from build123d import *

# Parameters (mm, degrees)
F0_W     = 15
F0_H     = 14
F0_R     = 3
F0_W_2   = 20
F0_H_2   = 2
F1_DEPTH = 2
F0_H_3   = 28
F0_W_3   = 12.9
F0_H_4   = 19.9
F2_DEPTH = 11.25
F3_R     = 5
F4_W     = 2
F4_H     = 1
F5_DEPTH = 2
F6_R     = 4.5
F6_R_2   = 2.75
F7_DEPTH = 9.25
F8_DEPTH = 2.001


with BuildPart() as f1:
    # F0 (on Top) → F1 (new body)
    with BuildSketch(Plane.XY):
        with Locations((-0.1896551724, 11.6551724138)):
            Rectangle(F0_W, F0_H)
        with Locations((-0.1896551724, 11.6551724138)):
            Circle(F0_R, mode=Mode.SUBTRACT)
        Polygon((-7.6896551724, 4.6551724138), (-22.6896551724, 4.6551724138), (-22.6896551724, 0.6551724138), (-9.1896551724, 0.6551724138), (10.8103448276, 0.6551724138), (24.3103448276, 0.6551724138), (24.3103448276, 4.6551724138), (7.3103448276, 4.6551724138), align=None)
        Polygon((-9.1896551724, 0.6551724138), (-22.6896551724, 0.6551724138), (-22.6896551724, -29.3448275862), (-9.1896551724, -29.3448275862), (-9.1896551724, -27.3448275862), align=None)
        Polygon((24.3103448276, 0.6551724138), (10.8103448276, 0.6551724138), (10.8103448276, -27.3448275862), (10.8103448276, -29.3448275862), (24.3103448276, -29.3448275862), align=None)
        with Locations((0.8103448276, -28.3448275862)):
            Rectangle(F0_W_2, F0_H_2)
    extrude(amount=F1_DEPTH)

    # F0 (on Top) → F2 (join)
    with BuildSketch(Plane.XY):
        with Locations((0.8103448276, -13.3448275862)):
            Rectangle(F0_W_2, F0_H_3)
        with Locations((0.8103448276, -15.3448275862)):
            Rectangle(F0_W_3, F0_H_4, mode=Mode.SUBTRACT)
    extrude(amount=F2_DEPTH)

    # F3
    f3_edges = [f1.edges().sort_by_distance(p)[0] for p in [
        (10.810345, 0.655172, 6.625),
        (-9.189655, 0.655172, 6.625),
        (-9.189655, -27.344828, 6.625),
        (10.810345, -27.344828, 6.625),
        (24.310345, -29.344828, 1),
        (-22.689655, -29.344828, 1),
        (24.310345, 4.655172, 1),
        (7.310345, 18.655172, 1),
        (-7.689655, 18.655172, 1),
        (-22.689655, 4.655172, 1),
        (-7.689655, 4.655172, 1),
        (7.310345, 4.655172, 1),
    ]]
    fillet(f3_edges, radius=F3_R)

    # F4 (on face) → F5 (cut)
    with BuildSketch(Plane(origin=(0, 0, 0), x_dir=(1, 0, 0), z_dir=(0, 0, -1))):
        with Locations((0.8603448276, 25.7948275862)):
            Rectangle(F4_W, F4_H)
        with Locations((0.8603448276, 4.8948275862)):
            Rectangle(F4_W, F4_H)
    extrude(amount=-F5_DEPTH, mode=Mode.SUBTRACT)

    # F6 (on face) → F7 (join)
    with BuildSketch(Plane.XY.offset(2)):
        with Locations((-15.6896551724, -23.3448275862)):
            Circle(F6_R)
        with Locations((-15.6896551724, -23.3448275862)):
            Circle(F6_R_2, mode=Mode.SUBTRACT)
        with Locations((17.3103448276, -23.3448275862)):
            Circle(F6_R)
        with Locations((17.3103448276, -23.3448275862)):
            Circle(F6_R_2, mode=Mode.SUBTRACT)
    extrude(amount=F7_DEPTH)

    # F8 (cut, through all): faces of the model
    f8_faces = [f1.faces().sort_by_distance(p)[0] for p in [
        (-15.6896551724, -23.3448275862, 2),
        (17.3103448276, -23.3448275862, 2),
    ]]
    extrude(f8_faces, amount=-F8_DEPTH, mode=Mode.SUBTRACT)


solid = f1.part
Build history of the part. All positions in model axes, mm. A direction names the side the tool comes from. Coordinates: 2 decimals unless noted, no trailing zeros. Order: outer loops, then holes, each group sorted by start corner. A loop starts at its lowest first (then second) coordinate and runs counter-clockwise, first axis right, second up. Notation, with made-up numbers: (44, 32) - (64, 32) arc R10 ccw to (64, 47) - close; hole circle Ø4 at (40.5, 16.25). An arc over 180 degrees is marked (long way). Write item = value, one per line. Start each with the question number.
1) Wall check: line 1 along X through (y, z) = (-7, 7); line 2 along X through (y, z) = (-15, 0.75); line 3 along X through (y, z) = (-23.5, 8.5). Give the ranges that are in metal, low to high. Write a range as from..to.
2) Saw through at B-B on y = -12.5. Write the cut outline in (x, z), then the cut area to 3 significant figures.
3) Saw through at A-A on z = 4. Write the cut outline in (x, y), then the cut area to 3 significant figures.
4) Saw through at D-D on y = 12.5. Write the cut outline in (x, z).
5) 3-axis set-ups, long thin cutter, end or side, ignore diameter. For faces 1 (the face through (-15, 4.655, 1)), 2 (the face through (-13.613, -27.337, 6.56)), 3 (the face through (-9.19, -13, 7)): which of +Z, -Z, +X, -X, +Y, -Y reach the whole face in a straight line?
6) Flat gauge pins, fed straight in: pin 1 Ø3.5 at (x, z) = (3, 7.5) entering from -Y; pin 2 Ø3.5 at (y, z) = (-17.5, 4.5) entering from -X; pin 3 Ø8 at (x, y) = (-0.19, 11.66) entering from +Z. Where does each tip first touch, or does it go through?
7) Two-plate mould, pull along X, no slides. Class faces 4 (the face through (1, -29.345, 1)), 5 (the face through (1, -25.295, 6)), 6 (the face through (7.31, 12, 1)): pulls with the +X half, pulls with the -X half, needs draft (parallel to the pull), parting line crosses it, or undercut.
8) Saw through at C-C on x = 16. Write the cut outline in (y, z).
From the geometry:
q1.line_1 = -9.19..-5.64, 7.26..10.81
q1.line_2 = -22.69..-5.64, 7.26..24.31
q1.line_3 = -20.19..-18.44, -12.94..-11.19, -9.05..-5.64, 7.26..10.68, 12.81..14.56, 20.06..21.81
q2.outline = (-22.69, 0) - (-5.64, 0) - (-5.64, 11.25) - (-9.19, 11.25) - (-9.19, 2) - (-22.69, 2) - close; (7.26, 0) - (24.31, 0) - (24.31, 2) - (10.81, 2) - (10.81, 11.25) - (7.26, 11.25) - close
q2.area = 134 mm^2
q3.outline = circle Ø9 at (-15.69, -23.34); (-9.19, -22.34) arc R5 ccw to (-4.19, -27.34) - (5.81, -27.34) arc R5 ccw to (10.81, -22.34) - (10.81, -4.34) arc R5 ccw to (5.81, 0.66) - (-4.19, 0.66) arc R5 ccw to (-9.19, -4.34) - close; circle Ø9 at (17.31, -23.34); hole circle Ø5.5 at (-15.69, -23.34); hole (-5.64, -25.29) - (7.26, -25.29) - (7.26, -5.39) - (-5.64, -5.39) - close; hole circle Ø5.5 at (17.31, -23.34)
q3.area = 362 mm^2
q4.outline = (-7.69, 0) - (-3.07, 0) - (-3.07, 2) - (-7.69, 2) - close; (2.69, 0) - (7.31, 0) - (7.31, 2) - (2.69, 2) - close
q5.face_1 = +Z, -Z, -X, +Y
q5.face_2 = +Z
q5.face_3 = +Z, +Y, -Y
q6.pin_1 = -27.34
q6.pin_2 = -17.56
q6.pin_3 = 2
q7.face_4 = needs draft
q7.face_5 = undercut
q7.face_6 = pulls with the +X half
q8.outline = (-29.34, 0) - (-25.76, 0) - (-25.76, 11.25) - (-27.65, 11.25) - (-27.65, 2) - (-29.34, 2) - close; (-20.93, 0) - (4.66, 0) - (4.66, 2) - (-19.04, 2) - (-19.04, 11.25) - (-20.93, 11.25) - close
